Here's the drawing with two shaded views (mm, measured from the low corner). I have some questions. Round coordinates to 2 decimals unless told otherwise and drop trailing zeros. Loops run counter-clockwise (first coordinate to the right, second up) from the corner with the lowest first, then second, coordinate; pieces in that order, holes last.
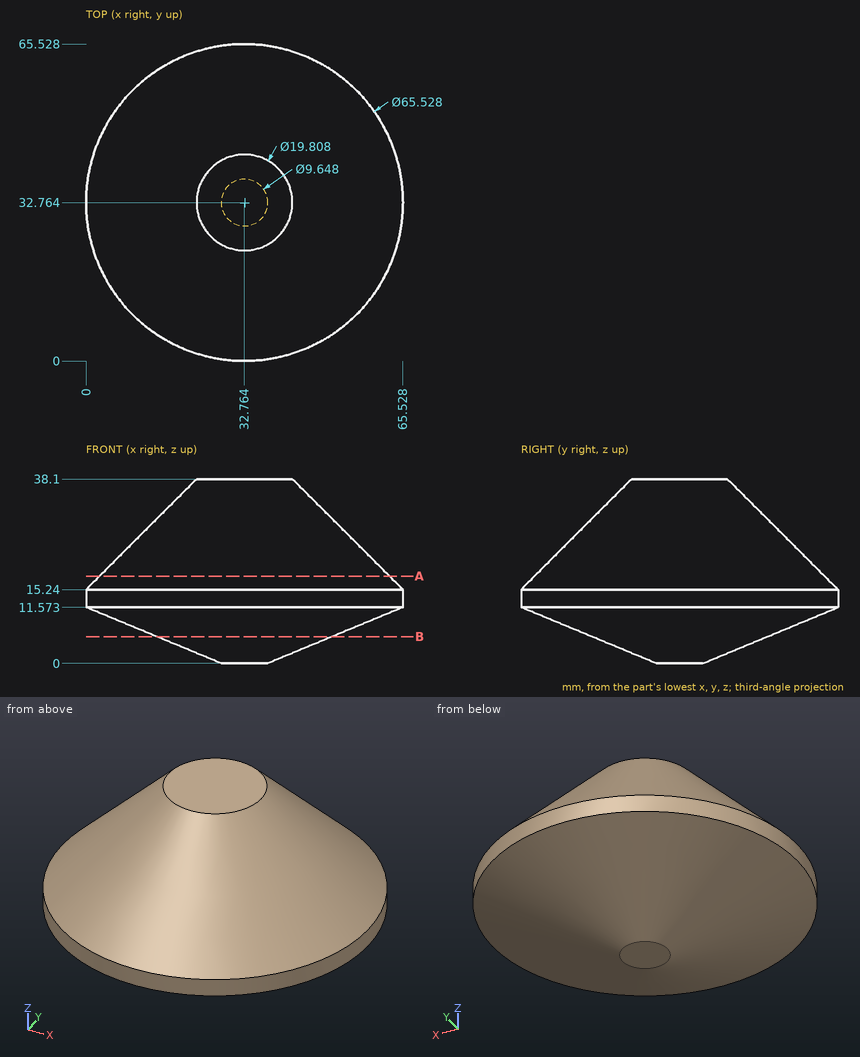
Item 1: Will these pins go through, and if not, where does the flat tip stop? pin 1 (12 mm diameter, centred on y = 17.5, z = 10, fed in from +X); pin 2 (12 mm diameter, centred on x = 47, y = 36, fed in from -Z); pin 3 (1 mm diameter, centred on y = 18.5, z = 22, fed in from +X).
Results list:
pin 1: stops at x = 64.13
pin 2: stops at z = 1.56
pin 3: stops at x = 55.18
Item 2: If we section it at B-B, the plane z = 5.5: Please give me the cut outline in (x, y), then the cut area to 3 significant figures.
Results list:
outline: circle Ø36.2 at (32.76, 32.76)
area: 1,030 mm2
Item 3: If we section it at A-A, the plane z = 18: Please give me the cut outline in (x, y).
Results list:
outline: circle Ø60.01 at (32.76, 32.76)
Item 4: If I drill on line 1 along Y through (x, z) = (20.5, 30.5) (1 decimal); line 2 along Z through (x, y) = (43, 15); line 3 along Z through (x, y) = (36, 44) (1 decimal), over which ranges is the centre line in solid material (lowest first)?
Results list:
line 1: y = 20.3 to 45.3
line 2: z = 6.49 to 27.5
line 3: z = 2.8 to 36.3
